Autodesk Inventor part; units mm, degrees
ref_plane "作業平面1" through (-4, 103.4, 0) normal (-1, 0, 0) x (0, -1, 0)
ref_plane "YZ Plane" through (0, 0, 0) normal (1, 0, 0) x (0, 1, 0)
ref_plane "XZ Plane" through (0, 0, 0) normal (0, 1, 0) x (-1, 0, 0)
sketch "スケッチ1" plane through (0, 0, 0) normal (0, 1, 0) x (-1, 0, 0)
  circle A0 centre (0, 0) radius 5
  dimension "d0" = 10
extrude "押し出し1" add sketch "スケッチ1" along normal blind 51.8
sketch "スケッチ2" plane through (0, 51.8, 0) normal (0, 1, 0) x (1, 0, 0)
  circle A0 centre (0, 0) radius 4
  dimension "d3" = 8
extrude "押し出し2" add sketch "スケッチ2" along normal blind 51.6
sketch "スケッチ3" plane through (0, 0, 0) normal (0, -1, 0) x (1, 0, 0)
  circle A0 centre (0, 0) radius 5
  circle A1 centre (0, 0) radius 4
  dimension "d6" = 8
extrude "押し出し3" add sketch "スケッチ3" along normal blind 43 contours A1
sketch "スケッチ4" plane through (0, 103.4, 0) normal (0, 1, 0) x (1, 0, 0)
  circle A0 centre (0, 0) radius 4
  point P0 (-4, 0)
ref_plane "作業平面1" through (-4, 103.4, 0) normal (-1, 0, 0) x (0, -1, 0)
sketch "スケッチ5" plane through (-4, 103.4, 0) normal (-1, 0, 0) x (0, -1, 0)
  line L0 (5, 1.5) -> (21, 1.5)
  line L1 (21, 1.5) -> (21, -1.5)
  line L2 (21, -1.5) -> (5, -1.5)
  line L3 (5, -1.5) -> (5, 1.5)
  line L4 (5, 1.5) -> (21, -1.5) construction
  line L5 (21, 1.5) -> (5, -1.5) construction
  line L6 (0, 4) -> (0, -4)
  point P0 (103.4, 0)
  point P1 (13, 0)
  dimension "d10" = 16
  dimension "d11" = 3
  dimension "d12" = 5
extrude "押し出し4" cut sketch "スケッチ5" against normal blind 1.8
sketch "スケッチ6" plane through (-4, 103.4, 0) normal (-1, 0, 0) x (0, -1, 0)
  line L0 (125.4, 1.5) -> (141.4, 1.5)
  line L1 (141.4, 1.5) -> (141.4, -1.5)
  line L2 (141.4, -1.5) -> (125.4, -1.5)
  line L3 (125.4, -1.5) -> (125.4, 1.5)
  line L4 (125.4, 1.5) -> (141.4, -1.5) construction
  line L5 (141.4, 1.5) -> (125.4, -1.5) construction
  line L6 (146.4, -4) -> (146.4, 4)
  point P0 (103.4, 0)
  point P1 (133.4, 0)
  dimension "d18" = 16
  dimension "d19" = 3
  dimension "d20" = 5
extrude "押し出し5" cut sketch "スケッチ6" against normal blind 1.8
properties part number "elbow_shaft" material "鋼、炭素鋼"
Design review of the part built by this model. Coordinates are the model's own, in mm. A direction names the side the tool comes from. Coordinates: 2 decimals unless noted, no trailing zeros. Write each loop counter-clockwise with the first axis right and the second up, starting at its lowest first coordinate (ties: lowest second). Pieces come first, ordered by that corner, then holes. Notation, with made-up numbers: M 1.25,19.25 L 47.25,19.25 A27 ccw 47.25,49.25 Z; hole C 67.5,83 d3. An arc over 180 degrees is marked long. Answer as a JSON object with one key per item and string values.
Item 1: Add section B-B, the plane z = 2.75. Give the boundary of the cut face in (x, y).
Outcome:
{"outline": "M -4.18,0 L -2.9,0 L -2.9,-43 L 2.9,-43 L 2.9,0 L 4.18,0 L 4.18,51.8 L 2.9,51.8 L 2.9,103.4 L -2.9,103.4 L -2.9,51.8 L -4.18,51.8 Z"}
Item 2: Wall thickness on probe 1 along Z at (x, y) = (-0.25, 40); probe 2 along Y at (x, z) = (1.75, 4.25): over which ranges is each line inside the solid? List them lowest first.
Outcome:
{"probe 1": "-4.99 to 4.99", "probe 2": "0 to 51.8"}
Item 3: Add section D-D, the plane y = 40. Give the boundary of the cut face in (x, z), and give its area (3 significant figures).
Outcome:
{"outline": "C 0,0 d10", "area": "78.5 mm²"}
Item 4: Draft analysis for pull direction Z (two halves, no side actions). For faces 1 (the cylindrical face through (3.695, 77.239, -1.532)), 2 (the flat face through (0, 103.4, 0)), 3 (the flat face through (-2.2, -30, 0)), state which applies: pulls with the +Z half, pulls with the -Z half, needs draft (parallel to the pull), parting line crosses it, or undercut.
Outcome:
{"face 1": "parting line crosses it", "face 2": "needs draft", "face 3": "undercut"}
Item 5: Machinability: for faces 4 (the flat face through (-2.2, 91, 0)), 5 (the cylindrical face through (3.695, -21.199, 1.532)), 6 (the cylindrical face through (1.08, 25.54, 4.88)), which of the approach directions +Z, -Z, +X, -X, +Y, -Y give a long, thin tool a straight path to every point of the face, cutting with its end or side? Answer none if there is none.
Outcome:
{"face 4": "-X", "face 5": "-Y", "face 6": "+Y, -Y"}
Item 6: Insertion check: pin 1 Ø1.7 at (x, y) = (-3, 87) entering from -Z; pin 2 Ø3.5 at (y, z) = (-33, 0.5) entering from -X; pin 3 Ø1 at (x, y) = (-3.5, 81) entering from +Z. Each pin has a flat end and moves straight along its axis. Give the tip position at first contact, or say it passes through.
Outcome:
{"pin 1": "z = -3.37", "pin 2": "x = -3.71", "pin 3": "z = 2.65"}
Item 7: Add section A-A, the plane x = 0. Give the boundary of the cut face in (y, z), and give its area (3 significant figures).
Outcome:
{"outline": "M -43,-4 L 0,-4 L 0,-5 L 51.8,-5 L 51.8,-4 L 103.4,-4 L 103.4,4 L 51.8,4 L 51.8,5 L 0,5 L 0,4 L -43,4 Z", "area": "1,270 mm²"}
Item 8: Add section C-C, the plane y = -25.5. Give the boundary of the cut face in (x, z), and give its area (3 significant figures).
Outcome:
{"outline": "M -3.71,-1.5 A4 ccw long -3.71,1.5 L -2.2,1.5 L -2.2,-1.5 Z", "area": "45.2 mm²"}
